from build123d import *

# Parameters (mm, degrees)
RESSALTO_EXTRUS_O1_DEPTH = 22.5
CHANFRO1_SIZE            = 9
CORTE_EXTRUS_O1_REACH    = 24.5
ESBO_O3_W                = 1139.230904301
ESBO_O3_H                = 709.798033895
CORTE_EXTRUS_O5_DEPTH    = 1.5
ESBO_O5_R                = 3
CORTE_EXTRUS_O6_DEPTH    = 22
CORTE_EXTRUS_O8_DEPTH    = 10
CORTE_EXTRUS_O9_DEPTH    = 22


with BuildPart() as part:
    # Esboço1 → Ressalto-extrusão1 (new body, symmetric)
    with BuildSketch(Plane.XY):
        with BuildLine():
            Line((-57.319579452, 11.917784657), (57.319579452, 11.917784657))
            Line((57.319579452, 11.917784657), (70, 22.557920862))
            Line((70, 22.557920862), (70, 117.296691049))
            ThreePointArc((70, 117.296691049), (70.546863139, 120.39810603), (72.121492792, 123.125444592))
            Line((72.121492792, 123.125444592), (112.878507208, 171.697762944))
            ThreePointArc((112.878507208, 171.697762944), (114.453136861, 174.425101506), (115, 177.526516487))
            Line((115, 177.526516487), (115, 237.712528581))
            ThreePointArc((115, 237.712528581), (114.396926208, 241.132730014), (112.660444431, 244.140404678))
            Line((112.660444431, 244.140404678), (75.567830361, 288.345660754))
            ThreePointArc((75.567830361, 288.345660754), (72.133568548, 290.980862527), (67.90738593, 291.917784657))
            Line((67.90738593, 291.917784657), (-67.90738593, 291.917784657))
            ThreePointArc((-67.90738593, 291.917784657), (-72.133568548, 290.980862527), (-75.567830361, 288.345660754))
            Line((-75.567830361, 288.345660754), (-112.660444431, 244.140404678))
            ThreePointArc((-112.660444431, 244.140404678), (-114.396926208, 241.132730014), (-115, 237.712528581))
            Line((-115, 237.712528581), (-115, 177.526516487))
            ThreePointArc((-115, 177.526516487), (-114.453136861, 174.425101506), (-112.878507208, 171.697762944))
            Line((-112.878507208, 171.697762944), (-72.121492792, 123.125444592))
            ThreePointArc((-72.121492792, 123.125444592), (-70.546863139, 120.39810603), (-70, 117.296691049))
            Line((-70, 117.296691049), (-70, 22.557920862))
            Line((-70, 22.557920862), (-57.319579452, 11.917784657))
        make_face()
        Polygon((-90, 175.546696324), (-90, 233.938676426), (-58.131744291, 271.917784657), (58.131744291, 271.917784657), (90, 233.938676426), (90, 175.546696324), (45, 121.917784657), (45, 31.917784657), (-45, 31.917784657), (-45, 121.917784657), align=None, mode=Mode.SUBTRACT)
    extrude(amount=RESSALTO_EXTRUS_O1_DEPTH, both=True)

    # Chanfro1
    chanfro1_edges = [part.edges().sort_by_distance(p)[0] for p in [
        (70, 69.927305955, 22.5),
        (70.546863139, 120.39810603, 22.5),
        (92.5, 147.411603768, 22.5),
        (114.453136861, 174.425101506, 22.5),
        (115, 207.619522534, 22.5),
        (114.396926208, 241.132730014, 22.5),
        (94.114137396, 266.243032716, 22.5),
        (72.133568548, 290.980862527, 22.5),
        (0, 291.917784657, 22.5),
        (-72.133568548, 290.980862527, 22.5),
        (-94.114137396, 266.243032716, 22.5),
        (-114.396926208, 241.132730014, 22.5),
        (-115, 207.619522534, 22.5),
        (-114.453136861, 174.425101506, 22.5),
        (-92.5, 147.411603768, 22.5),
        (-70.546863139, 120.39810603, 22.5),
        (-70, 69.927305955, 22.5),
        (-63.659789726, 17.23785276, 22.5),
        (0, 11.917784657, 22.5),
        (63.659789726, 17.23785276, 22.5),
    ]]
    chamfer(chanfro1_edges, length=CHANFRO1_SIZE)

    # Esboço3 → Corte-extrusão1 (cut, up to next)
    with BuildSketch(Plane.XY, mode=Mode.PRIVATE) as corte_extrus_o1_sk1:
        with Locations((-153.157436203, 152.53565808)):
            Rectangle(ESBO_O3_W, ESBO_O3_H)
    corte_extrus_o1_tool1 = extrude(corte_extrus_o1_sk1.sketch, amount=-CORTE_EXTRUS_O1_REACH, mode=Mode.PRIVATE) & part.part
    add(corte_extrus_o1_tool1.solids().sort_by_distance((-153.157436, 152.535658, 0))[0], mode=Mode.SUBTRACT)

    # Esboço4 → Corte-extrusão5 (cut)
    with BuildSketch(Plane.XY.offset(22.5)):
        Polygon((-60, 27.220997444), (-53.679877109, 21.917784657), (53.679877109, 21.917784657), (60, 27.220997444), (60, 125.792574104), (105, 179.421485771), (105, 237.712528581), (67.90738593, 281.917784657), (-67.90738593, 281.917784657), (-105, 237.712528581), (-105, 179.421485771), (-60, 125.792574104), align=None)
        Polygon((-90, 175.546696324), (-90, 233.938676426), (-58.131744291, 271.917784657), (58.131744291, 271.917784657), (90, 233.938676426), (90, 175.546696324), (45, 121.917784657), (45, 31.917784657), (-45, 31.917784657), (-45, 121.917784657), align=None, mode=Mode.SUBTRACT)
    extrude(amount=-CORTE_EXTRUS_O5_DEPTH, mode=Mode.SUBTRACT)

    # Esboço5 → Corte-extrusão6 (cut, through all)
    with BuildSketch(Plane.XY.offset(21)):
        with Locations((-93, 244)):
            Circle(ESBO_O5_R)
        with Locations((-52.5, 60.396230411)):
            Circle(ESBO_O5_R)
        with Locations((-72, 266.917784657)):
            Circle(ESBO_O5_R)
        with Locations((-52.5, 36.917784657)):
            Circle(ESBO_O5_R)
        with Locations((52.5, 36.917784657)):
            Circle(ESBO_O5_R)
        with Locations((72, 266.917784657)):
            Circle(ESBO_O5_R)
        with Locations((52.5, 60.396230411)):
            Circle(ESBO_O5_R)
        with Locations((93, 244)):
            Circle(ESBO_O5_R)
    extrude(amount=-CORTE_EXTRUS_O6_DEPTH, mode=Mode.SUBTRACT)

    # Esboço7 → Corte-extrusão8 (cut)
    with BuildSketch(Plane(origin=(0, 0, 0), x_dir=(-1, 0, 0), z_dir=(0, 0, -1))):
        Polygon((-73.109400392, 271.401372964), (-76.43760157, 268.198809887), (-75.328201177, 263.715221581), (-70.890599608, 262.434196351), (-67.56239843, 265.636759427), (-68.671798823, 270.120347733), align=None)
        Polygon((-92.305785489, 247.981381613), (-96.100870363, 246.591898209), (-96.795084874, 242.610516596), (-93.694214511, 240.018618387), (-89.899129637, 241.408101791), (-89.204915126, 245.389483404), align=None)
        Polygon((93, 248.041451884), (89.5, 246.020725942), (89.5, 241.979274058), (93, 239.958548116), (96.5, 241.979274058), (96.5, 246.020725942), align=None)
        Polygon((72.832050294, 270.280475887), (69.503849117, 269.319706964), (68.671798823, 265.957015734), (71.167949706, 263.555093427), (74.496150883, 264.51586235), (75.328201177, 267.87855358), align=None)
        Polygon((-52.5, 64.437682295), (-56, 62.416956353), (-56, 58.375504468), (-52.5, 56.354778526), (-49, 58.375504468), (-49, 62.416956353), align=None)
        Polygon((52.5, 64.437682295), (49, 62.416956353), (49, 58.375504468), (52.5, 56.354778526), (56, 58.375504468), (56, 62.416956353), align=None)
        Polygon((52.5, 40.959236541), (49, 38.938510599), (49, 34.897058715), (52.5, 32.876332773), (56, 34.897058715), (56, 38.938510599), align=None)
        Polygon((-51.54604516, 40.845036049), (-55.424122052, 39.707559479), (-56.378076893, 35.780308087), (-53.45395484, 32.990533265), (-49.575877948, 34.128009835), (-48.621923107, 38.055261227), align=None)
    extrude(amount=-CORTE_EXTRUS_O8_DEPTH, mode=Mode.SUBTRACT)

    # Esboço8 → Corte-extrusão9 (cut, through all)
    with BuildSketch(Plane.XY.offset(21)):
        Polygon((-105, 237.712528581), (-90, 233.938676426), (-90, 175.546696324), (-45, 121.917784657), (-60, 125.792574104), (-105, 179.421485771), align=None)
        Polygon((90, 233.938676426), (105, 237.712528581), (105, 179.421485771), (60, 125.792574104), (45, 121.917784657), (90, 175.546696324), align=None)
    extrude(amount=-CORTE_EXTRUS_O9_DEPTH, mode=Mode.SUBTRACT)


solid = part.part
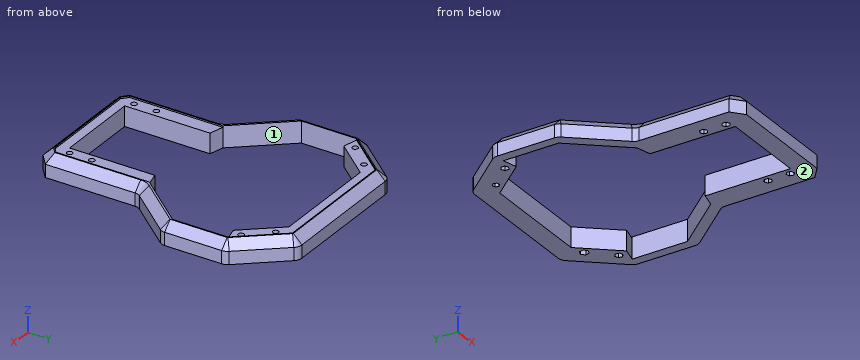
Can you work these out from the model? Positions are in its coordinate system, mm. Face numbers are marked on the shaded views. Coordinates: 2 decimals unless noted, no trailing zeros. Write each loop counter-clockwise with the first axis right and the second up, starting at its lowest first coordinate (ties: lowest second). Pieces come first, ordered by that corner, then holes. Notation, with made-up numbers: (15, -7) -> (45, -7) arc R26 cw to (45, 10) -> close; hole circle Ø1 at (57.25, 27.25). An arc over 180 degrees is marked (long way). Write each question's results on one line, items separated by ' | '. Start each with the question number.
Q1. We'd pull the mould along Y, two halves only. Please class the marked faces 1 and 2: +Y half, -Y half, draft (parallel to the pull), parting line (faces both ways), or undercut.
Q2. Imagine slicing it at D-D (y = 193). Write out the boundary of the cut face in (x, z).
Q3. If I drill on probe 1 along Y at (x, z) = (72, 12); probe 2 along X at (y, z) = (183.5, 9.75); probe 3 along X at (y, z) = (96.5, 1.75), over which ranges is the centre line in solid material (lowest first)?
Q4. Imagine slicing it at B-B (z = 6.25). State how many separate pieces and enclosed holes the cut face has, then the cut area to 3 significant figures.
Q5. Imagine slicing it at C-C (x = -81.5). Write out the boundary of the cut face in (y, z).
Q6. Imagine slicing it at A-A (y = 109). Write out the boundary of the cut face in (x, z).
Q7. I'm going to push flat-ended pins straight in: pin 1 (2 mm diameter, centred on y = 146.5, z = 10, fed in from -X); pin 2 (2 mm diameter, centred on y = 134, z = 15, fed in from -X); pin 3 (10 mm diameter, centred on x = 60.5, y = 261, fed in from -Z); pin 4 (1.3 mm diameter, centred on x = -71.5, y = 264.5, fed in from -Z). Where does each tip first touch, or does it pass through?
Taken from the geometry:
1) face 1: undercut | face 2: draft
2) outline: (-115, 0) -> (-105, 0) -> (-105, 22.5) -> (-106, 22.5) -> (-115, 13.5) -> close; (105, 0) -> (115, 0) -> (115, 13.5) -> (106, 22.5) -> (105, 22.5) -> close
3) probe 1: y = 122.98 to 140.09, 255.39 to 263.92, 269.92 to 291.04 | probe 2: x = -115 to -105, 105 to 115 | probe 3: x = -70 to -45, 45 to 70
4) separate pieces: 1 | enclosed holes: 9 | area: 15,100 mm^2
5) outline: (134.3, 0) -> (151.42, 0) -> (151.42, 22.5) -> (148.3, 22.5) -> (134.3, 13.5) -> close; (244.07, 0) -> (281.28, 0) -> (281.28, 13.5) -> (267.27, 22.5) -> (265.72, 22.5) -> (265.72, 21) -> (244.07, 21) -> close
6) outline: (-70, 0) -> (-45, 0) -> (-45, 21) -> (-60, 21) -> (-60, 22.5) -> (-61, 22.5) -> (-70, 13.5) -> close; (45, 0) -> (70, 0) -> (70, 13.5) -> (61, 22.5) -> (60, 22.5) -> (60, 21) -> (45, 21) -> close
7) pin 1: stops at x = -92.57 | pin 2: stops at x = -80.84 | pin 3: passes through | pin 4: stops at z = 10
